Answer from the drawing. Dimensions are ordinates in mm from the lowest x, y and z of the part. Round coordinates to 2 decimals unless told otherwise and drop trailing zeros. Write each loop counter-clockwise with the first axis right and the second up, starting at its lowest first coordinate (ties: lowest second). Pieces come first, ordered by that corner, then holes. Notation, with made-up numbers: (-17, 60) - (16, 60) arc R16 cw to (16, 71) - close; hole circle Ø4 at (-38.5, -21.5). An arc over 180 degrees is marked (long way). One line per item, written item: value. Start each with the question number.
(1) A cutting plane is placed at D-D, the plane z = 3. Determine the outline of the cut face in (x, y), plus the area to 3 significant figures.
(2) Find the intervals of material crossed by L1, parallel to Y at x = 9.25, z = 20.75; L2, parallel to Z at x = 9.75, y = 14, in increasing order.
(3) A cutting plane is placed at A-A, the plane y = 9.25. Determine the outline of the cut face in (x, z), plus the area to 4 significant figures.
(4) Flat-ended cylindrical pins translate along their axes: pin 1 Ø3.5 at (x, y) = (9.25, 9.25) entering from -Z; pin 2 Ø8 at (y, z) = (14, 19.5) entering from +X; pin 3 Ø1 at (x, z) = (15.5, 12) entering from -Y; pin 4 Ø3 at (x, z) = (13, 23.5) entering from +Y. Find the tip coordinate at first contact, or state that the pin passes through.
(5) The mould has two halves that part along X. Classify the marked faces 1, 2 and 3: +X half, -X half, draft (parallel to the pull), parting line (faces both ways), or undercut.
(6) A cutting plane is placed at C-C, the plane z = 10. Determine the outline of the cut face in (x, y), plus the area to 3 significant figures.
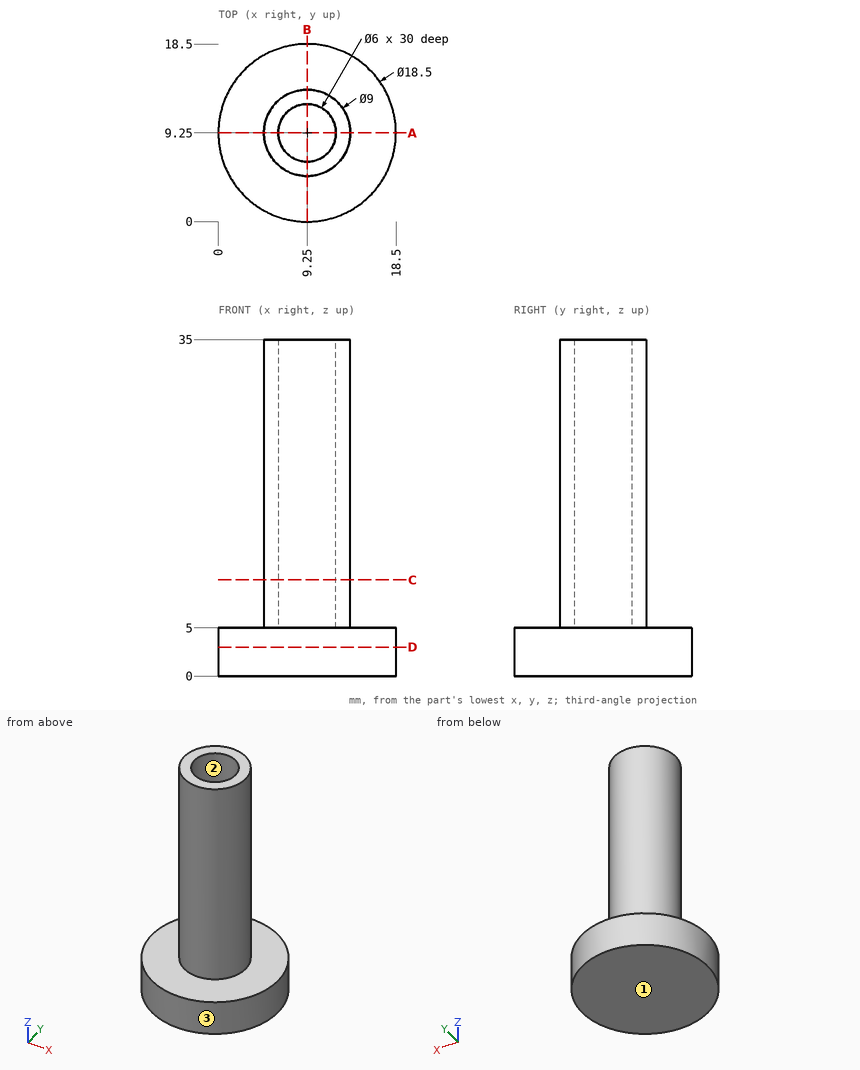
Here are the results:
1. outline: circle Ø18.5 at (9.25, 9.25)
1. area: 269 mm²
2. L1: 4.75 to 6.25, 12.25 to 13.75
2. L2: 0 to 5
3. outline: (0, 0) - (18.5, 0) - (18.5, 5) - (13.75, 5) - (13.75, 35) - (12.25, 35) - (12.25, 5) - (6.25, 5) - (6.25, 35) - (4.75, 35) - (4.75, 5) - (0, 5) - close
3. area: 182.5 mm²
4. pin 1: z = 0
4. pin 2: x = 13.69
4. pin 3: through
4. pin 4: y = 13.15
5. face 1: draft
5. face 2: undercut
5. face 3: parting line
6. outline: circle Ø9 at (9.25, 9.25); hole circle Ø6 at (9.25, 9.25)
6. area: 35.3 mm²
